```python
from build123d import *

# Parameters (mm, degrees)
F0_W     = 118.589319
F0_H     = 162.553676
F1_DEPTH = 25.4
F2_R     = 5.08
F3_T     = -2.54


with BuildPart() as f1:
    # F0 (on Top) → F1 (new body)
    with BuildSketch(Plane.XY):
        with Locations((59.294659, 57.971325)):
            Rectangle(F0_W, F0_H)
    extrude(amount=F1_DEPTH)

    # F2
    f2_edges = [f1.edges().sort_by_distance(p)[0] for p in [
        (118.589319, -23.305513, 12.7),
        (118.589319, 139.248163, 12.7),
        (0, 139.248163, 12.7),
        (0, -23.305513, 12.7),
    ]]
    fillet(f2_edges, radius=F2_R)

    # F3
    f3_openings = [f1.faces().sort_by_distance(p)[0] for p in [
        (59.29466, 57.971325, 25.4),
    ]]
    offset(amount=F3_T, openings=f3_openings)


solid = f1.part
```
Verification items for the finished model (mm, model axes). A direction names the side the tool comes from. Round coordinates to 2 decimals unless told otherwise and drop trailing zeros. Write each loop counter-clockwise with the first axis right and the second up, starting at its lowest first coordinate (ties: lowest second). Pieces come first, ordered by that corner, then holes.
1. Section check C-C on y = 93.5. Enter the section's corners in (x, z), plus the area to 3 significant figures.
2. Draft check along Y on faces 3 (the flat face through (2.54, 57, 14)), 4 (the flat face through (118.589, 57, 13)), 5 (the cylindrical face through (117.06, -21.86, 12.88)). Enter one of: +Y half, -Y half, draft (parallel to the pull), parting line (faces both ways), or undercut.
3. Section check A-A on x = 77. Enter the section's corners in (y, z), plus the area to 3 significant figures.
4. Access from +Z, -Z, +X, -X, +Y, -Y to the whole of each face (thin tool, end or side, straight path). Record for faces 1 (the flat face through (59, -23.306, 13)), 2 (the flat face through (59, 59, 2.54)).
5. Section check B-B on z = 16.25. Enter the section's corners in (x, y).
6. Scan lines: L1, parallel to Y at x = 38.5, z = 10; L2, parallel to X at y = 90.5, z = 19; L3, parallel to Z at x = 91, y = 67. Record each from-to range of solid material in increasing order.
Answer:
1. outline: (0, 0) - (118.59, 0) - (118.59, 25.4) - (116.05, 25.4) - (116.05, 2.54) - (2.54, 2.54) - (2.54, 25.4) - (0, 25.4) - close
1. area: 417 mm2
2. face 3: undercut
2. face 4: draft
2. face 5: -Y half
3. outline: (-23.31, 0) - (139.25, 0) - (139.25, 25.4) - (136.71, 25.4) - (136.71, 2.54) - (-20.77, 2.54) - (-20.77, 25.4) - (-23.31, 25.4) - close
3. area: 529 mm2
4. face 1: +Z, -Z, +X, -X, -Y
4. face 2: +Z
5. outline: (0, -18.23) arc R5.08 ccw to (5.08, -23.31) - (113.51, -23.31) arc R5.08 ccw to (118.59, -18.23) - (118.59, 134.17) arc R5.08 ccw to (113.51, 139.25) - (5.08, 139.25) arc R5.08 ccw to (0, 134.17) - close; hole (2.54, -18.23) arc R2.54 ccw to (5.08, -20.77) - (113.51, -20.77) arc R2.54 ccw to (116.05, -18.23) - (116.05, 134.17) arc R2.54 ccw to (113.51, 136.71) - (5.08, 136.71) arc R2.54 ccw to (2.54, 134.17) - close
6. L1: y = -23.31 to -20.77, 136.71 to 139.25
6. L2: x = 0 to 2.54, 116.05 to 118.59
6. L3: z = 0 to 2.54
